Geometry: see drawing. Coordinates: mm, zero at the bounding-box minimum. A direction names the side the tool comes from. Give positions to 0.01 mm unless a question says otherwise; leave off trailing zeros. Write each loop counter-clockwise with the first axis right and the second up, starting at its lowest first coordinate (ties: lowest second). Pieces come first, ordered by that corner, then holes. Notation, with made-up numbers: (14.25, -22.5) - (45.25, -22.5) arc R21 cw to (45.25, -9.5) - close; hole circle Ø1 at (-1.75, 31.25). An arc over 180 degrees is marked (long way). Return JSON: item names as keys, results as strings.
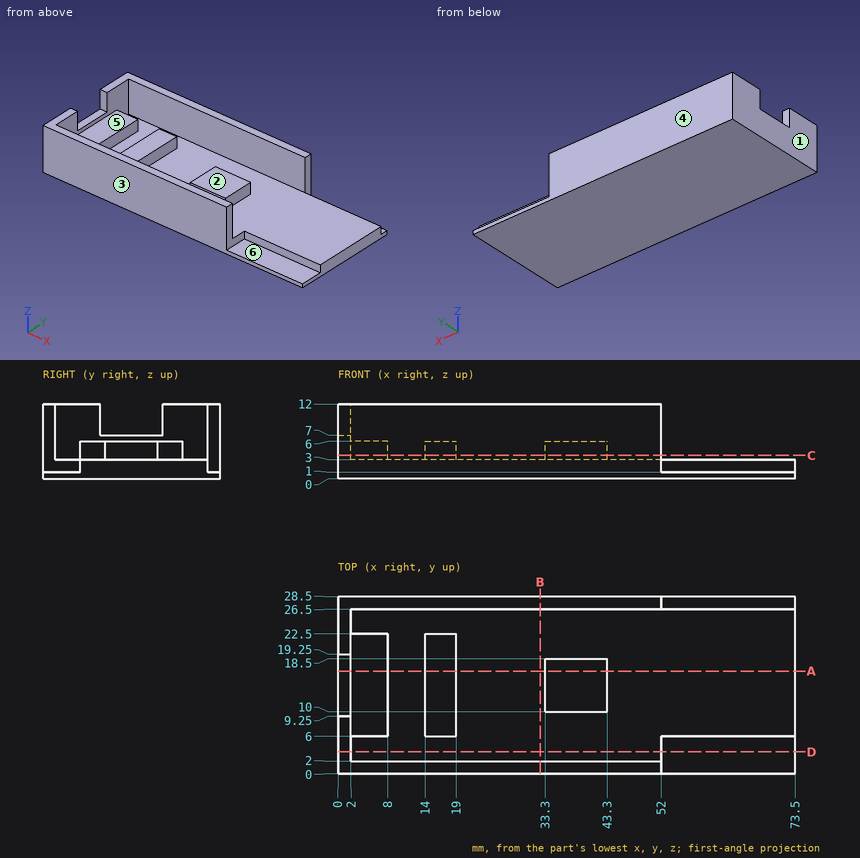
Q1. Pin query (flat end, axial travel): P1, Ø2.5, axis at x = 16, y = 14.5, coming from the +Z side; P2, Ø3.5, axis at y = 13.5, z = 5, coming from the +X side; P3, Ø1, axis at x = 62.5, z = 2, coming from the +Y side. Return the tip coordinate at first contact, or that it passes through.
Answer key:
{"P1": "stops at z = 6", "P2": "stops at x = 43.3", "P3": "stops at y = 26.5"}
Q2. Section query D-D, the plane y = 3.5. Return the cut outline in (x, z), plus the area to 4 significant figures.
Answer key:
{"outline": "(0, 0) - (73.5, 0) - (73.5, 1) - (52, 1) - (52, 3) - (2, 3) - (2, 12) - (0, 12) - close", "area": "195.5 mm^2"}
Q3. Section query C-C, the plane z = 3.75. Return the cut outline in (x, y), plus the area to 4 significant figures.
Answer key:
{"outline": "(0, 0) - (52, 0) - (52, 2) - (2, 2) - (2, 6) - (8, 6) - (8, 22.5) - (2, 22.5) - (2, 26.5) - (52, 26.5) - (52, 28.5) - (0, 28.5) - close; (14, 6) - (19, 6) - (19, 22.5) - (14, 22.5) - close; (33.3, 10) - (43.3, 10) - (43.3, 18.5) - (33.3, 18.5) - close", "area": "523.5 mm^2"}
Q4. Section query A-A, the plane y = 16.5. Return the cut outline in (x, z), plus the area to 4 significant figures.
Answer key:
{"outline": "(0, 0) - (73.5, 0) - (73.5, 3) - (43.3, 3) - (43.3, 6) - (33.3, 6) - (33.3, 3) - (19, 3) - (19, 6) - (14, 6) - (14, 3) - (8, 3) - (8, 6) - (2, 6) - (2, 7) - (0, 7) - close", "area": "291.5 mm^2"}
Q5. Material intervals for probe 1 along Y at (x, z) = (37, 4); probe 2 along X at (y, z) = (16.75, 3.25); probe 3 along X at (y, z) = (21, 5.25), sorted ascending. Write a range as [from, to].
Answer key:
{"probe 1": "y = [0, 2], [10, 18.5], [26.5, 28.5]", "probe 2": "x = [0, 8], [14, 19], [33.3, 43.3]", "probe 3": "x = [0, 8], [14, 19]"}
Q6. Section query B-B, the plane x = 32.5. Return the cut outline in (y, z), plus the area to 4 significant figures.
Answer key:
{"outline": "(0, 0) - (28.5, 0) - (28.5, 12) - (26.5, 12) - (26.5, 3) - (2, 3) - (2, 12) - (0, 12) - close", "area": "121.5 mm^2"}
Q7. Set-up query: the marked faces 4, 5 and 6. Return all of +Z, -Z, +X, -X, +Y, -Y with unobstructed straight access to the full face (end or side cutting, diameter ignored); none if empty.
Answer key:
{"face 4": "+Z, -Z, +X, -X, +Y", "face 5": "+Z, +X", "face 6": "+Z, +X, -Y"}
Q8. Mould query, pull axis Y, two halves, no side actions, for the marked faces 1, 2 and 3. Classes: pulls with the +Y half, pulls with the -Y half, needs draft (parallel to the pull), parting line crosses it, or undercut.
Answer key:
{"face 1": "needs draft", "face 2": "undercut", "face 3": "pulls with the -Y half"}
